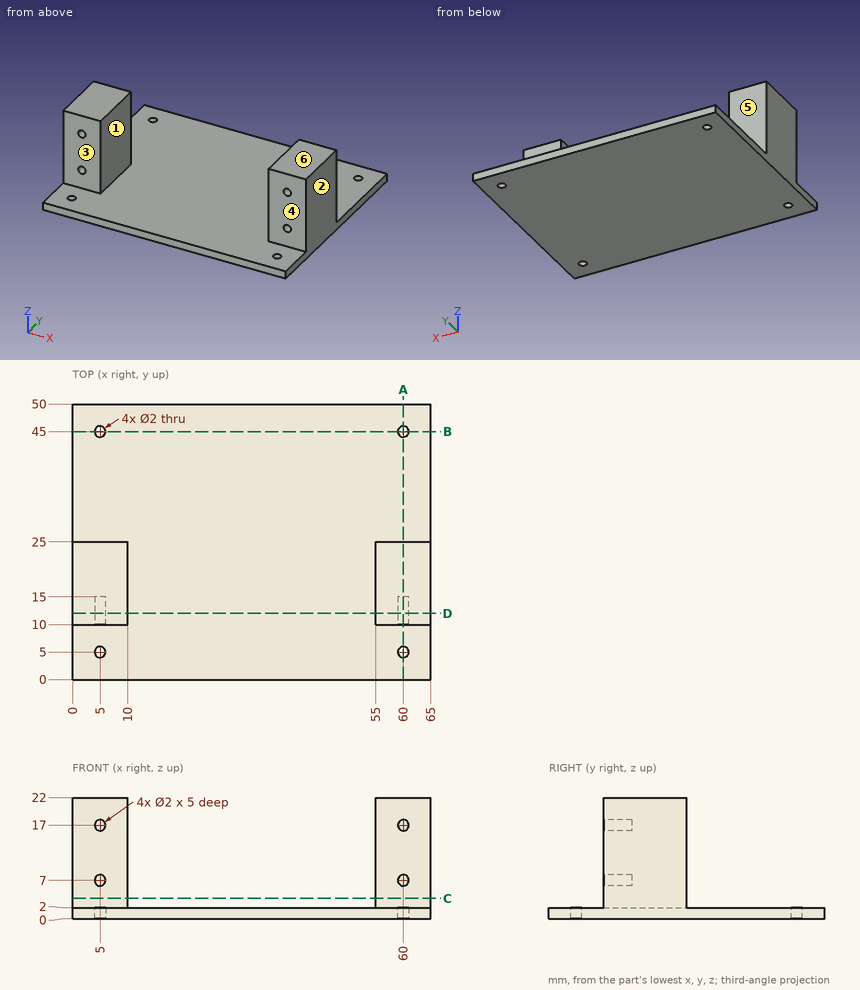
Part print with two shaded views. Sizes in mm from the minimum x, y, z corner. A direction names the side the tool comes from. Round coordinates to 2 decimals unless told otherwise and drop trailing zeros. Loops run counter-clockwise (first coordinate to the right, second up) from the corner with the lowest first, then second, coordinate; pieces in that order, holes last. Notation, with made-up numbers: M -35.75,33 L 3.25,33 A28 ccw 3.25,58 Z; hole C 34.25,17 d4. An arc over 180 degrees is marked long. Return JSON: item names as keys, results as strings. Group by question number.
(1) Saw through at A-A, the plane x = 60. List the corners of the cut face in (y, z).
(2) Drop flat-ended pins along their axis: P1, Ø8, axis at x = 59, z = 11.5, coming from the +Y side; P2, Ø2.5, axis at x = 60, y = 45, coming from the +Z side; P3, Ø1.6, axis at x = 5, z = 6.5, coming from the -Y side. Give the stop position or say it passes through.
(3) Saw through at C-C, the plane z = 3.75. List the corners of the cut face in (x, y), and give its area (3 significant figures).
(4) Saw through at D-D, the plane y = 12. List the corners of the cut face in (x, z), and give its area (3 significant figures).
(5) Tool access for the marked faces 4, 5 and 6: list every direction of +Z, -Z, +X, -X, +Y, -Y with a clear straight run to the whole face (end or side of a thin tool).
(6) Mould opens along X. For the marked faces 1, 2 and 3 say: +X half, -X half, draft (parallel to the pull), parting line (faces both ways), or undercut.
(7) Saw through at B-B, the plane y = 45. List the corners of the cut face in (x, z).
(8) Wall check: probe 1 along Z at (x, y) = (60, 13.95); probe 2 along Y at (x, z) = (60, 1.3); probe 3 along X at (y, z) = (23, 17.5). Give the ranges that are in metal, low to high. Write a range as [from, to].
Answer list:
{
 "1": {"outline": "M 0,0 L 4,0 L 4,2 L 0,2 Z; M 6,0 L 44,0 L 44,2 L 25,2 L 25,22 L 10,22 L 10,18 L 15,18 L 15,16 L 10,16 L 10,8 L 15,8 L 15,6 L 10,6 L 10,2 L 6,2 Z; M 46,0 L 50,0 L 50,2 L 46,2 Z"},
 "2": {"P1": "y = 25", "P2": "z = 2", "P3": "y = 10"},
 "3": {"outline": "M 0,10 L 10,10 L 10,25 L 0,25 Z; M 55,10 L 65,10 L 65,25 L 55,25 Z", "area": "300 mm2"},
 "4": {"outline": "M 0,0 L 65,0 L 65,22 L 55,22 L 55,2 L 10,2 L 10,22 L 0,22 Z; hole C 5,7 d2; hole C 5,17 d2; hole C 60,7 d2; hole C 60,17 d2", "area": "517 mm2"},
 "5": {"face 4": "+Z, +X, -X, -Y", "face 5": "+Z, +X, -X, +Y", "face 6": "+Z, +X, -X, +Y, -Y"},
 "6": {"face 1": "undercut", "face 2": "+X half", "face 3": "draft"},
 "7": {"outline": "M 0,0 L 4,0 L 4,2 L 0,2 Z; M 6,0 L 59,0 L 59,2 L 6,2 Z; M 61,0 L 65,0 L 65,2 L 61,2 Z"},
 "8": {"probe 1": "[0, 6], [8, 16], [18, 22]", "probe 2": "[0, 4], [6, 44], [46, 50]", "probe 3": "[0, 10], [55, 65]"}
}
